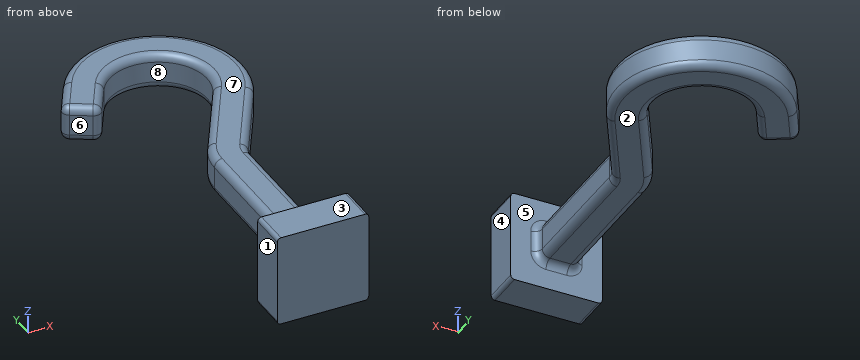
```python
from build123d import *

# Parameters (mm, degrees)
SKETCH1_W           = 24
SKETCH1_H           = 24
BOSS_EXTRUDE1_DEPTH = 10
FILLET1_R           = 2
FILLET2_R           = 1


with BuildPart() as part:
    # Sketch1 → Boss-Extrude1 (new body)
    with BuildSketch(Plane(origin=(0, 0, 0), x_dir=(1, 0, 0), z_dir=(0, 1, 0))):
        Rectangle(SKETCH1_W, SKETCH1_H)
    extrude(amount=BOSS_EXTRUDE1_DEPTH)

    # Sweep1: sweep along a path in Sketch2
    with BuildLine(Plane.XY) as sweep1_path:
        Line((0, 10), (0, 46.32050807568873))
        ThreePointArc((0, 46.32050807568873), (0.3407417371093189, 48.90869852671398), (1.3397459621556382, 51.320508075688814))
        Line((1.3397459621556382, 51.320508075688814), (13.500000000000028, 72.38268590217983))
        ThreePointArc((13.500000000000028, 72.38268590217983), (7.094555433772385, 96.28813046840753), (-16.810889132455312, 89.88268590217987))
        Line((-16.810889132455312, 89.88268590217987), (-22.310889132455326, 80.35640646055106))
    # Sketch3 → Sweep1 (sweep)
    with BuildSketch(Plane(origin=(0, 10, 0), x_dir=(1, 0, 0), z_dir=(0, 1, 0))):
        with BuildLine():
            Line((2.7499999999999853, -4.750000000000002), (-2.749999999999986, -4.750000000000001))
            ThreePointArc((-2.749999999999986, -4.750000000000001), (-4.164213562373095, -4.164213562373096), (-4.75, -2.7499999999999867))
            Line((-4.75, -2.7499999999999867), (-4.75, 2.7499999999999853))
            ThreePointArc((-4.75, 2.7499999999999853), (-4.164213562373094, 4.164213562373095), (-2.7499999999999853, 4.749999999999999))
            Line((-2.7499999999999853, 4.749999999999999), (2.7499999999999862, 4.749999999999998))
            ThreePointArc((2.7499999999999862, 4.749999999999998), (4.164213562373096, 4.164213562373094), (4.750000000000001, 2.749999999999984))
            Line((4.750000000000001, 2.749999999999984), (4.75, -2.749999999999987))
            ThreePointArc((4.75, -2.749999999999987), (4.164213562373096, -4.164213562373097), (2.7499999999999853, -4.750000000000002))
        make_face()
    sweep(path=sweep1_path.line)

    # Fillet1
    fillet1_edges = [part.edges().sort_by_distance(p)[0] for p in [
        (-18.704574400656547, 78.27429967936449, 4.164213562373096),
        (-22.310889132455365, 80.35640646055109, 4.750000000000002),
        (-25.91720386425412, 82.43851324173762, 4.164213562373098),
        (-26.42450980043141, 82.73140646055109, 1.78e-15),
        (-25.917203864254123, 82.43851324173762, -4.164213562373092),
        (-22.310889132455365, 80.35640646055109, -4.749999999999998),
        (-18.704574400656547, 78.27429967936449, -4.164213562373094),
        (-18.197268464479265, 77.98140646055103, 8.9e-16),
        (-4.4e-16, 10, 4.750000000000002),
        (4.164213562373095, 10, 4.164213562373098),
        (4.75, 10, 1.78e-15),
        (4.164213562373097, 10, -4.164213562373092),
        (4.4e-16, 10, -4.749999999999998),
        (-4.164213562373095, 10, -4.164213562373094),
        (-4.75, 10, 8.9e-16),
        (-4.164213562373096, 10, 4.164213562373096),
    ]]
    fillet(fillet1_edges, radius=FILLET1_R)

    # Fillet2
    fillet2_edges = [part.edges().sort_by_distance(p)[0] for p in [
        (12, 5, 12),
        (-12, 5, 12),
        (-12, 5, -12),
        (12, 5, -12),
    ]]
    fillet(fillet2_edges, radius=FILLET2_R)


solid = part.part
```
For this review, take the finished solid that the model builds, in its own axes (mm). Face numbers are marked on the shaded views. A direction names the side the tool comes from. Round coordinates to 2 decimals unless told otherwise and drop trailing zeros. Write each loop counter-clockwise with the first axis right and the second up, starting at its lowest first coordinate (ties: lowest second). Pieces come first, ordered by that corner, then holes. Notation, with made-up numbers: M 62,78 L 110,78 A27 cw 110,100 Z; hole C 84.5,-7.5 d11. An arc over 180 degrees is marked long. One line per item, written item: value. Start each with the question number.
(1) Machinability: for the marked faces 1, 2, 3, 4 and 5, which of the approach directions +Z, -Z, +X, -X, +Y, -Y give a long, thin tool a straight path to every point of the face, cutting with its end or side? Answer none if there is none.
(2) We need section C-C (z = 9.75). Give the boundary of the cut face in (x, y).
(3) Insertion check: pin 1 (8 mm diameter, centred on y = 4.5, z = -4.5, fed in from +X); pin 2 (12 mm diameter, centred on x = 7.5, y = 24.5, fed in from -Z); pin 3 (12 mm diameter, centred on x = -7.5, y = 62.5, fed in from -Z); pin 4 (3 mm diameter, centred on y = 87, z = -6, fed in from -X). Each pin has a flat end and moves straight along its axis. Give the tip position at first contact, or say it passes through.
(4) Wall thickness on line 1 (Y direction, x = 4, z = 9.75); line 2 (X direction, y = 18, z = 1.5); line 3 (X direction, y = 91.5, z = -2.5): over which ranges is each line inside the solid? List them lowest first.
(5) We need section A-A (y = 42). Give the boundary of the cut face in (x, z), and give its area (3 significant figures).
(6) The part is to be moulded in two halves that separate along Y. For the marked faces 6, 7 and 8, say which applies: released by +Y, released by -Y, zero draft, split by the parting line, or undercut.
Result:
1. face 1: +Z, -Z, -X, -Y
1. face 2: -Z, +X, -X, +Y
1. face 3: +Z, +X, -X, +Y, -Y
1. face 4: +Z, -Z, +X, -Y
1. face 5: none
2. outline: M -12,0 L 12,0 L 12,10 L -12,10 Z
3. pin 1: x = 12
3. pin 2: z = -4.75
3. pin 3: through
3. pin 4: x = -22.88
4. line 1: 0 to 10
4. line 2: -4.75 to 4.75
4. line 3: -21.36 to -9.08, 5.77 to 18.03
5. outline: M -4.75,-2.75 A2 ccw -2.75,-4.75 L 2.75,-4.75 A2 ccw 4.75,-2.75 L 4.75,2.75 A2 ccw 2.75,4.75 L -2.75,4.75 A2 ccw -4.75,2.75 Z
5. area: 86.8 mm²
6. face 6: released by -Y
6. face 7: zero draft
6. face 8: undercut
